Verification items for the finished model (mm, model axes). A direction names the side the tool comes from. Round coordinates to 2 decimals unless told otherwise and drop trailing zeros. Order: outer loops, then holes, each group sorted by start corner. A loop starts at its lowest first (then second) coordinate and runs counter-clockwise, first axis right, second up. Notation, with made-up numbers: (-22, 16) -> (-18, 16) arc R26 cw to (-18, 48) -> close; hole circle Ø11 at (62.5, 19.5). An arc over 180 degrees is marked (long way). Put each result on its own line as item: value.
from build123d import *

# Parameters (mm, degrees)
SKETCH2_W               = 1000
SKETCH2_H               = 1000
BOSS_EXTRUDE1_DEPTH     = 100
SKETCH3_W               = 800
SKETCH3_H               = 800
BOSS_EXTRUDE2_DEPTH     = 100
SKETCH4_W               = 600
SKETCH4_H               = 600
BOSS_EXTRUDE3_DEPTH     = 100
SKETCH5_W               = 400
SKETCH5_H               = 400
BOSS_EXTRUDE4_DEPTH     = 100
SKETCH6_W               = 200
SKETCH6_H               = 200
BOSS_EXTRUDE5_DEPTH     = 100
CUT_EXTRUDE2_DEPTH      = 1470.69384567
CUT_EXTRUDE2_DEPTH_BACK = 1470.69384567
SKETCH8_W               = 250
SKETCH8_H               = 250
CUT_EXTRUDE3_DEPTH      = 1519.222645069
CUT_EXTRUDE3_DEPTH_BACK = 70
SKETCH17_W              = 200
SKETCH17_H              = 200
BOSS_EXTRUDE6_DEPTH     = 100
SKETCH18_W              = 100
SKETCH18_H              = 100
BOSS_EXTRUDE7_DEPTH     = 100
SKETCH19_W              = 25
SKETCH19_H              = 25
BOSS_EXTRUDE8_DEPTH     = 100
SKETCH20_W              = 50
SKETCH20_H              = 50
BOSS_EXTRUDE9_DEPTH     = 100
SKETCH21_R              = 50
CUT_EXTRUDE4_DEPTH      = 10
SKETCH22_R              = 25
CUT_EXTRUDE5_DEPTH      = 10


with BuildPart() as part:
    # Sketch2 → Boss-Extrude1 (new body)
    with BuildSketch(Plane(origin=(0, 0, 0), x_dir=(1, 0, 0), z_dir=(0, 1, 0))):
        with Locations((500, 500)):
            Rectangle(SKETCH2_W, SKETCH2_H)
    extrude(amount=BOSS_EXTRUDE1_DEPTH)

    # Sketch3 → Boss-Extrude2 (add)
    with BuildSketch(Plane(origin=(0, 100, 0), x_dir=(1, 0, 0), z_dir=(0, 1, 0))):
        with Locations((500, 500)):
            Rectangle(SKETCH3_W, SKETCH3_H)
    extrude(amount=BOSS_EXTRUDE2_DEPTH)

    # Sketch4 → Boss-Extrude3 (add)
    with BuildSketch(Plane(origin=(0, 200, 0), x_dir=(1, 0, 0), z_dir=(0, 1, 0))):
        with Locations((500, 500)):
            Rectangle(SKETCH4_W, SKETCH4_H)
    extrude(amount=BOSS_EXTRUDE3_DEPTH)

    # Sketch5 → Boss-Extrude4 (add)
    with BuildSketch(Plane(origin=(0, 300, 0), x_dir=(1, 0, 0), z_dir=(0, 1, 0))):
        with Locations((500, 500)):
            Rectangle(SKETCH5_W, SKETCH5_H)
    extrude(amount=BOSS_EXTRUDE4_DEPTH)

    # Sketch6 → Boss-Extrude5 (add)
    with BuildSketch(Plane(origin=(0, 400, 0), x_dir=(1, 0, 0), z_dir=(0, 1, 0))):
        with Locations((500, 500)):
            Rectangle(SKETCH6_W, SKETCH6_H)
    extrude(amount=BOSS_EXTRUDE5_DEPTH)

    # Sketch8 → Cut-Extrude2 (cut, two sides: drawn at the far end of the back side and taken through both)
    with BuildSketch(Plane(origin=(0, 100, 0), x_dir=(1, 0, 0), z_dir=(0, 1, 0)).offset(-CUT_EXTRUDE2_DEPTH_BACK)):
        with Locations((125, 125)):
            Rectangle(SKETCH8_W, SKETCH8_H)
        with Locations((875, 125)):
            Rectangle(SKETCH8_W, SKETCH8_H)
        with Locations((875, 875)):
            Rectangle(SKETCH8_W, SKETCH8_H)
        with Locations((125, 875)):
            Rectangle(SKETCH8_W, SKETCH8_H)
    extrude(amount=CUT_EXTRUDE2_DEPTH + CUT_EXTRUDE2_DEPTH_BACK, mode=Mode.SUBTRACT)

    # Sketch16 → Cut-Extrude3 (cut, two sides: drawn at the far end of the back side and taken through both)
    with BuildSketch(Plane(origin=(0, 50, 50), x_dir=(1, 0, 0), z_dir=(0, 0.7071067811865477, 0.7071067811865475)).offset(-CUT_EXTRUDE3_DEPTH_BACK)):
        Polygon((450, 636.396103068), (450, -32.366607249), (540.963803132, -32.366607249), (550, 636.396103068), align=None)
    extrude(amount=CUT_EXTRUDE3_DEPTH + CUT_EXTRUDE3_DEPTH_BACK, mode=Mode.SUBTRACT)

    # Sketch17 → Boss-Extrude6 (add)
    with BuildSketch(Plane(origin=(0, 0, 0), x_dir=(1, 0, 0), z_dir=(0, 1, 0))):
        with Locations((150, 850)):
            Rectangle(SKETCH17_W, SKETCH17_H)
        with Locations((850, 850)):
            Rectangle(SKETCH17_W, SKETCH17_H)
        with Locations((850, 150)):
            Rectangle(SKETCH17_W, SKETCH17_H)
        with Locations((150, 150)):
            Rectangle(SKETCH17_W, SKETCH17_H)
    extrude(amount=BOSS_EXTRUDE6_DEPTH)

    # Sketch18 → Boss-Extrude7 (add)
    with BuildSketch(Plane(origin=(0, 100, 0), x_dir=(1, 0, 0), z_dir=(0, 1, 0))):
        with Locations((200, 200)):
            Rectangle(SKETCH18_W, SKETCH18_H)
        with Locations((800, 200)):
            Rectangle(SKETCH18_W, SKETCH18_H)
        with Locations((800, 800)):
            Rectangle(SKETCH18_W, SKETCH18_H)
        with Locations((200, 800)):
            Rectangle(SKETCH18_W, SKETCH18_H)
    extrude(amount=BOSS_EXTRUDE7_DEPTH)

    # Sketch19 → Boss-Extrude8 (add)
    with BuildSketch(Plane(origin=(0, 200, 0), x_dir=(1, 0, 0), z_dir=(0, 1, 0))):
        with Locations((762.5, 237.5)):
            Rectangle(SKETCH19_W, SKETCH19_H)
        with Locations((762.5, 762.5)):
            Rectangle(SKETCH19_W, SKETCH19_H)
        with Locations((237.5, 762.5)):
            Rectangle(SKETCH19_W, SKETCH19_H)
        with Locations((237.5, 237.5)):
            Rectangle(SKETCH19_W, SKETCH19_H)
    extrude(amount=BOSS_EXTRUDE8_DEPTH)

    # Sketch20 → Boss-Extrude9 (add)
    with BuildSketch(Plane(origin=(0, 500, 0), x_dir=(1, 0, 0), z_dir=(0, 1, 0))):
        with Locations((425, 575)):
            Rectangle(SKETCH20_W, SKETCH20_H)
        with Locations((425, 425)):
            Rectangle(SKETCH20_W, SKETCH20_H)
        with Locations((575, 425)):
            Rectangle(SKETCH20_W, SKETCH20_H)
        with Locations((575, 575)):
            Rectangle(SKETCH20_W, SKETCH20_H)
    extrude(amount=BOSS_EXTRUDE9_DEPTH)

    # Sketch21 → Cut-Extrude4 (cut)
    with BuildSketch(Plane(origin=(0, 500, 0), x_dir=(1, 0, 0), z_dir=(0, 1, 0))):
        with Locations(Location((500, 500, 0), (0, 0, 270))):
            Circle(SKETCH21_R)
    extrude(amount=-CUT_EXTRUDE4_DEPTH, mode=Mode.SUBTRACT)

    # Sketch22 → Cut-Extrude5 (cut)
    with BuildSketch(Plane(origin=(0, 400, 0), x_dir=(1, 0, 0), z_dir=(0, 1, 0))):
        with Locations(Location((350, 650, 0), (0, 0, 270))):
            Circle(SKETCH22_R)
        with Locations(Location((650, 650, 0), (0, 0, 90))):
            Circle(SKETCH22_R)
        with Locations(Location((650, 350, 0), (0, 0, 270))):
            Circle(SKETCH22_R)
        with Locations(Location((350, 350, 0), (0, 0, 90))):
            Circle(SKETCH22_R)
    extrude(amount=-CUT_EXTRUDE5_DEPTH, mode=Mode.SUBTRACT)


solid = part.part
Item 1: Tool access check on faces 1 (the cylindrical face through (640.42, 395.07, -326.91)), 2 (the flat face through (50, 49, -149)), 3 (the flat face through (950, 49, -149)), 4 (the flat face through (450, 549, -575)). Record the directions out of +Z, -Z, +X, -X, +Y, -Y that give a thin tool (end or side, any length) a straight path to the whole face; none if there is none.
Check sheet entries:
face 1: +Y
face 2: +Z, -X, +Y, -Y
face 3: +Z, +X, +Y, -Y
face 4: +Z, -Z, +Y
Item 2: Section check C-C on y = 266. Record the boundary of the cut face in (x, z), then the cut area to 3 significant figures.
Check sheet entries:
outline: (200, -750) -> (225, -750) -> (225, -775) -> (250, -775) -> (250, -800) -> (750, -800) -> (750, -775) -> (775, -775) -> (775, -750) -> (800, -750) -> (800, -250) -> (775, -250) -> (775, -225) -> (750, -225) -> (750, -200) -> (545.85, -200) -> (546.47, -264.99) -> (450, -264.99) -> (450, -200) -> (250, -200) -> (250, -225) -> (225, -225) -> (225, -250) -> (200, -250) -> close
area: 346,000 mm^2
Item 3: Section check D-D on z = -500. Record the boundary of the cut face in (x, y), then the cut area to 3 significant figures.
Check sheet entries:
outline: (0, 0) -> (1000, 0) -> (1000, 100) -> (900, 100) -> (900, 200) -> (800, 200) -> (800, 300) -> (700, 300) -> (700, 400) -> (600, 400) -> (600, 500) -> (550, 500) -> (550, 490) -> (450, 490) -> (450, 500) -> (400, 500) -> (400, 400) -> (300, 400) -> (300, 300) -> (200, 300) -> (200, 200) -> (100, 200) -> (100, 100) -> (0, 100) -> close
area: 299,000 mm^2
Item 4: Material ranges on L1, parallel to X at y = 393.75, z = -650; L2, parallel to X at y = 495, z = -500; L3, parallel to Z at x = 575.5, y = 566, recorded low to high. Write a range as [from, to].
Check sheet entries:
L1: x = [300, 325], [375, 625], [675, 700]
L2: x = [400, 450], [550, 600]
L3: z = [-600, -550], [-450, -400]
Item 5: Section check A-A on z = -829.5. Record the boundary of the cut face in (x, y).
Check sheet entries:
outline: (50, 0) -> (950, 0) -> (950, 100) -> (850, 100) -> (850, 200) -> (150, 200) -> (150, 100) -> (50, 100) -> close
Item 6: Gauge pin test, flat ends, axial feed: pin 1 Ø4 at (x, y) = (300.5, 326.5) entering from -Z; pin 2 Ø20 at (y, z) = (262, -217) entering from -X; pin 3 Ø15 at (x, y) = (868, 149.5) entering from -Z; pin 4 Ø12 at (x, z) = (680, -245) entering from -Y. Record the tip position at first contact, or that the pin passes through.
Check sheet entries:
pin 1: stops at z = -700
pin 2: stops at x = 225
pin 3: stops at z = -750
pin 4: stops at y = 0
